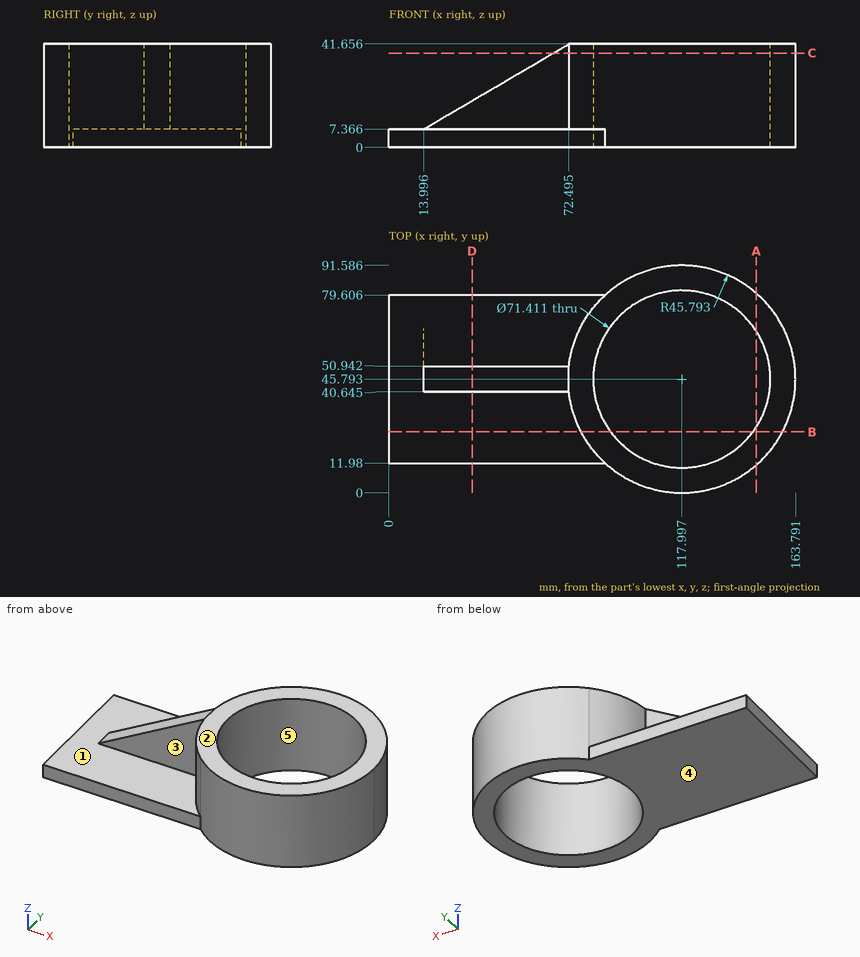
For this review, use the dimensioned drawing (mm, ordinates from the lowest corner) and the shaded views. A direction names the side the tool comes from. Coordinates: 2 decimals unless noted, no trailing zeros. Write each loop counter-clockwise with the first axis right and the second up, starting at its lowest first coordinate (ties: lowest second). Pieces come first, ordered by that corner, then holes. Notation, with made-up numbers: (-33, 82) - (6, 82) arc R29 cw to (6, 117) - close; hole circle Ø10 at (-4.75, 7.25). An arc over 180 degrees is marked (long way). Answer in a Markdown table with one row per item. Add a question column.
Q1. Consider section B-B on y = 24.5. Give the boundary of the cut face in (x, z) (1 decimal).
Q2. Consider section C-C on z = 38. Give the boundary of the cut face in (x, y) (1 decimal).
Q3. Consider section A-A on x = 148. Give the boundary of the cut face in (y, z) (1 decimal).
Q4. Consider section D-D on x = 33.5. Give the boundary of the cut face in (y, z) (1 decimal).
Q5. Draft analysis for pull direction Y (two halves, no side actions). For the marked faces 3, 4 and 5, state which applies: +Y half, -Y half, draft (parallel to the pull), parting line (faces both ways), or undercut.
Q6. Clearance check with flat-ended pins moving along their axes: pin 1 (17 mm diameter, centred on x = 48, z = 27.5, fed in from -Y) (1 decimal); pin 2 (2 mm diameter, centred on y = 59, z = 33, fed in from -X); pin 3 (8 mm diameter, centred on x = 100, z = 21, fed in from +Y) (1 decimal). State where each tip first meets the part, or that it passes through.
Q7. To check wall thickness, follow line 1 along Y through (x, z) = (69.5, 12.5) (1 decimal); line 2 along Y through (x, z) = (91.5, 33) (1 decimal); line 3 along Z through (x, y) = (71.5, 20.5). State the ranges of each line that lie inside material, in increasing order. Write a range as from..to.
Q8. For the marked faces 1 and 2, list the 3-axis set-ups (+Z, -Z, +X, -X, +Y, -Y) from which the entire face can be reached by the end or side of a thin tool; tool diameter is ignored.
Answers below:
| question | item | result |
|---|---|---|
| 1 | outline | (0, 0) - (89.3, 0) - (89.3, 41.7) - (77.5, 41.7) - (77.5, 7.4) - (0, 7.4) - close; (146.7, 0) - (158.5, 0) - (158.5, 41.7) - (146.7, 41.7) - close |
| 2 | outline | (66.3, 40.6) - (72.5, 40.6) arc R45.8 ccw (long way) to (72.5, 50.9) - (66.3, 50.9) - close; hole circle Ø71.4 at (118, 45.8) |
| 3 | outline | (11.2, 0) - (26.4, 0) - (26.4, 41.7) - (11.2, 41.7) - close; (65.2, 0) - (80.4, 0) - (80.4, 41.7) - (65.2, 41.7) - close |
| 4 | outline | (12, 0) - (79.6, 0) - (79.6, 7.4) - (50.9, 7.4) - (50.9, 18.8) - (40.6, 18.8) - (40.6, 7.4) - (12, 7.4) - close |
| 5 | face 3 | -Y half |
| 5 | face 4 | draft |
| 5 | face 5 | undercut |
| 6 | pin 1 | y = 40.6 |
| 6 | pin 2 | x = 73.86 |
| 6 | pin 3 | y = 89.4 |
| 7 | line 1 | 40.6..50.9 |
| 7 | line 2 | 8.4..21.9, 69.7..83.1 |
| 7 | line 3 | 0..7.37 |
| 8 | face 1 | +Z, -X |
| 8 | face 2 | +Z, +X, -X, +Y, -Y |
